```python
from build123d import *

# Parameters (mm, degrees)
SKETCH2_R           = 3
BOSS_EXTRUDE1_DEPTH = 40.6


with BuildPart() as part:
    # Sketch2 → Boss-Extrude1 (new body)
    with BuildSketch(Plane(origin=(0, 0, 0), x_dir=(0, 0, -1), z_dir=(1, 0, 0))):
        Polygon((10.969655115, 0), (5.484827557, 9.5), (-5.484827557, 9.5), (-10.969655115, 0), (-5.484827557, -9.5), (5.484827557, -9.5), align=None)
        Circle(SKETCH2_R, mode=Mode.SUBTRACT)
    extrude(amount=-BOSS_EXTRUDE1_DEPTH)

    # Sketch3 → Cut-Revolve1 (revolve, cut)
    with BuildSketch(Plane.XY, mode=Mode.PRIVATE) as cut_revolve1_sk:
        Polygon((-21.6, 9.5), (-21.6, 5.8), (-17.6, 5.8), (-16.55, 4.75), (-15.15, 4.75), (-14.1, 5.8), (-12.6, 5.8), (-11.55, 4.75), (-2.060608065, 4.75), (0, 4), (0, 12), (-22.269872981, 12), align=None)
        Polygon((-40.6, 9.5), (-40.6, 13), (-39.662177826, 13), align=None)
    revolve(cut_revolve1_sk.sketch.rotate(Axis((-40.6, 0, 0), (1, 0, 0)), 180), axis=Axis((-40.6, 0, 0), (1, 0, 0)), mode=Mode.SUBTRACT)

    # Sketch6 → 1/4 NPT Tapped Hole1 (revolve, cut)
    with BuildSketch(Plane(origin=(-40.6, 0, 0), x_dir=(0, 0, 1), z_dir=(0, 1, 0))):
        Polygon((0, 0), (0, 14.2), (5.5626, 14.2), (5.5626, 12), (6.56760783, 12), (6.9172709, 0.3217291), (7.239, 0), align=None)
    revolve(axis=Axis((-46.95, 0, 0), (1, 0, 0)), mode=Mode.SUBTRACT)


solid = part.part
```
CAD build for the part. Positions are in the model's coordinates, mm. A direction names the side the tool comes from. Coordinates: 2 decimals unless noted, no trailing zeros. Loops run counter-clockwise (first coordinate to the right, second up) from the corner with the lowest first, then second, coordinate; pieces in that order, holes last. Notation, with made-up numbers: (78, -29) - (129, -29) arc R13 cw to (129, -17) - close; hole circle Ø2 at (-2, 87.5). An arc over 180 degrees is marked (long way). Return JSON: item names as keys, results as strings.
1. Band-saw the part on B-B (x = -7). Give the cut face in (y, z).
Result:
{"outline": "circle Ø9.5 at (0, 0); hole circle Ø6 at (0, 0)"}
2. Band-saw the part on D-D (x = -29.5). Give the cut face in (y, z).
Result:
{"outline": "(-9.5, -5.48) - (0, -10.97) - (9.5, -5.48) - (9.5, 5.48) - (0, 10.97) - (-9.5, 5.48) - close; hole circle Ø13.19 at (0, 0)"}
3. Band-saw the part on C-C (x = -21). Give the cut face in (y, z).
Result:
{"outline": "circle Ø11.6 at (0, 0); hole circle Ø6 at (0, 0)"}
4. Band-saw the part on A-A (x = -36.5). Give the cut face in (y, z), and give its area (3 significant figures).
Result:
{"outline": "(-9.5, -5.48) - (0, -10.97) - (9.5, -5.48) - (9.5, 5.48) - (0, 10.97) - (-9.5, 5.48) - close; hole circle Ø13.61 at (0, 0)", "area": "167 mm2"}
5. Mould opens along Y. For faces 1 (the cylindrical face through (-27.515, -1.671, 5.306)), 2 (the cylindrical face through (-13.34, -5.532, -1.742)), 3 (the flat face through (-31, -4.8, -8.2)), 4 (the flat face through (-31, 9.5, 0)) say: released by +Y, released by -Y, zero draft, split by the parting line, or undercut.
Result:
{"face 1": "undercut", "face 2": "split by the parting line", "face 3": "released by -Y", "face 4": "released by +Y"}
6. Drop flat-ended pins along their axis: pin 1 (3 mm diameter, centred on x = -18, z = -3, fed in from +Y); pin 2 (2 mm diameter, centred on x = -28, y = 5, fed in from +Z); pin 3 (2 mm diameter, centred on y = -3.5, z = -2.5, fed in from -X). Give the stop position or say it passes through.
Result:
{"pin 1": "stops at y = 5.6", "pin 2": "stops at z = 8.66", "pin 3": "stops at x = -26.4"}
7. Probe L1, parallel to Z at x = -27.35, y = 0; L2, parallel to X at y = 1.25, z = 3.5; L3, parallel to X at y = 5, z = -6. List the from-to ranges inside material, lowest first. Write a range as from..to.
Result:
{"L1": "z = -10.97..-5.56, 5.56..10.97", "L2": "x = -26.4..0", "L3": "x = -40.6..-21.6"}
8. 3-axis set-ups, long thin cutter, end or side, ignore diameter. For faces 5 (the cylindrical face through (-13, 0, 3)), 6 (the flat face through (-21.6, -4.1, -4.4)): which of +Z, -Z, +X, -X, +Y, -Y reach the whole face in a straight line?
Result:
{"face 5": "+X, -X", "face 6": "+X"}
